The listing builds one solid part. Answer for the finished solid, in the listing's coordinates (mm). Face numbers are marked on the shaded views. A direction names the side the tool comes from. Round coordinates to 2 decimals unless told otherwise and drop trailing zeros. Write each loop counter-clockwise with the first axis right and the second up, starting at its lowest first coordinate (ties: lowest second). Pieces come first, ordered by that corner, then holes. Notation, with made-up numbers: (70.5, 72) - (83.5, 72) arc R12 cw to (83.5, 91) - close; hole circle Ø5 at (-5.5, 6.5). An arc over 180 degrees is marked (long way). Return JSON: item names as keys, results as strings. Group by question number.
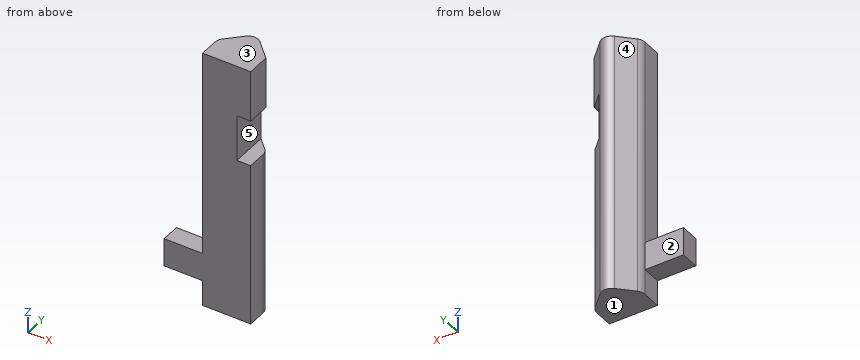
from build123d import *

# Parameters (mm, degrees)
SZKIC1_W                    = 9.4
SZKIC1_H                    = 4.5
DODANIE_WYCI_GNI_CIE1_DEPTH = 51
SZKIC2_W                    = 2.7
SZKIC2_H                    = 9
SZKIC2_W_2                  = 5.3
WYTNIJ_WYCI_GNI_CIE1_DEPTH  = 10
ZAOKR_GLENIE1_R             = 2
SZKIC5_W                    = 7.5
SZKIC5_H                    = 5.5
DODANIE_WYCI_GNI_CIE4_DEPTH = 3.67157


with BuildPart() as part:
    # Szkic1 → Dodanie-wyciągnięcie1 (new body)
    with BuildSketch(Plane.XY):
        Polygon((0, 6.95), (4.7, 2.25), (-4.7, 2.25), align=None)
        Rectangle(SZKIC1_W, SZKIC1_H)
    extrude(amount=DODANIE_WYCI_GNI_CIE1_DEPTH)

    # Szkic2 → Wytnij-wyciągnięcie1 (cut)
    with BuildSketch(Plane.XZ.offset(2.25)):
        with Locations((3.35, 36.5)):
            Rectangle(SZKIC2_W, SZKIC2_H)
        with Locations((7.35, 36.5)):
            Rectangle(SZKIC2_W_2, SZKIC2_H)
    extrude(amount=-WYTNIJ_WYCI_GNI_CIE1_DEPTH, mode=Mode.SUBTRACT)

    # Zaokrąglenie1
    zaokr_glenie1_edges = [part.edges().sort_by_distance(p)[0] for p in [
        (-4.7, 2.25, 25.5),
        (0, 6.95, 25.5),
        (4.7, 2.25, 16),
    ]]
    fillet(zaokr_glenie1_edges, radius=ZAOKR_GLENIE1_R)

    # Szkic5 → Dodanie-wyciągnięcie4 (add)
    with BuildSketch(Plane.XZ.offset(2.25)):
        with Locations((-8.45, 7.75)):
            Rectangle(SZKIC5_W, SZKIC5_H)
    extrude(amount=-DODANIE_WYCI_GNI_CIE4_DEPTH)


solid = part.part
(1) Determine the mould class of the marked faces 3, 4 and 5 for opening direction Z: +Z half, -Z half, draft (parallel to the pull), parting line (faces both ways), or undercut.
(2) Flat-ended cylindrical pins translate along their axes: pin 1 (1 mm diameter, centred on y = 5, z = 37.5, fed in from +X); pin 2 (6 mm diameter, centred on x = -7, z = 42, fed in from -Y); pin 3 (3 mm diameter, centred on x = -10, z = 8, fed in from +Y); pin 4 (1.8 mm diameter, centred on x = -8.5, y = -1, fed in from +Z). Find the tip coordinate at first contact, or state that the pin passes through.
(3) Find section A-A (z = 21). Write down the section's boundary in (x, y).
(4) Find section B-B (y = 0). Write down the section's boundary in (x, z), plus the area to 3 significant figures.
(5) Find section C-C (x = -8.5). Write down the section's boundary in (y, z).
(6) Consider line 1 (Z direction, x = 2.25, y = 3.25); line 2 (Z direction, x = -5, y = 0); line 3 (X direction, y = -1, z = 43). Determine where each line is inside the solid, lowest interval first.
(7) Find section D-D (z = 39.5). Write down the section's boundary in (x, y).
(8) For the marked faces 1 and 2, determine the directions among +Z, -Z, +X, -X, +Y, -Y from which every point of the face is accessible in a straight line to the end or side of a thin tool.
Check sheet entries:
{
 "1": {"face 3": "+Z half", "face 4": "draft", "face 5": "undercut"},
 "2": {"pin 1": "stops at x = 2", "pin 2": "stops at y = -2.25", "pin 3": "stops at y = 1.42", "pin 4": "stops at z = 10.5"},
 "3": {"outline": "(-4.7, -2.25) - (4.7, -2.25) - (4.7, 1.42) arc R2 ccw to (4.11, 2.84) - (1.41, 5.54) arc R2 ccw to (-1.41, 5.54) - (-4.11, 2.84) arc R2 ccw to (-4.7, 1.42) - close"},
 "4": {"outline": "(-12.2, 5) - (-4.7, 5) - (-4.7, 0) - (4.7, 0) - (4.7, 32) - (2, 32) - (2, 41) - (4.7, 41) - (4.7, 51) - (-4.7, 51) - (-4.7, 10.5) - (-12.2, 10.5) - close", "area": "496 mm^2"},
 "5": {"outline": "(-2.25, 5) - (1.42, 5) - (1.42, 10.5) - (-2.25, 10.5) - close"},
 "6": {"line 1": "z = 0 to 32, 41 to 51", "line 2": "z = 5 to 10.5", "line 3": "x = -4.7 to 4.7"},
 "7": {"outline": "(-4.7, -2.25) - (2, -2.25) - (2, 4.95) - (1.41, 5.54) arc R2 ccw to (-1.41, 5.54) - (-4.11, 2.84) arc R2 ccw to (-4.7, 1.42) - close"},
 "8": {"face 1": "-Z, +X, -X, +Y, -Y", "face 2": "+Z, -Z, -X, +Y"}
}
